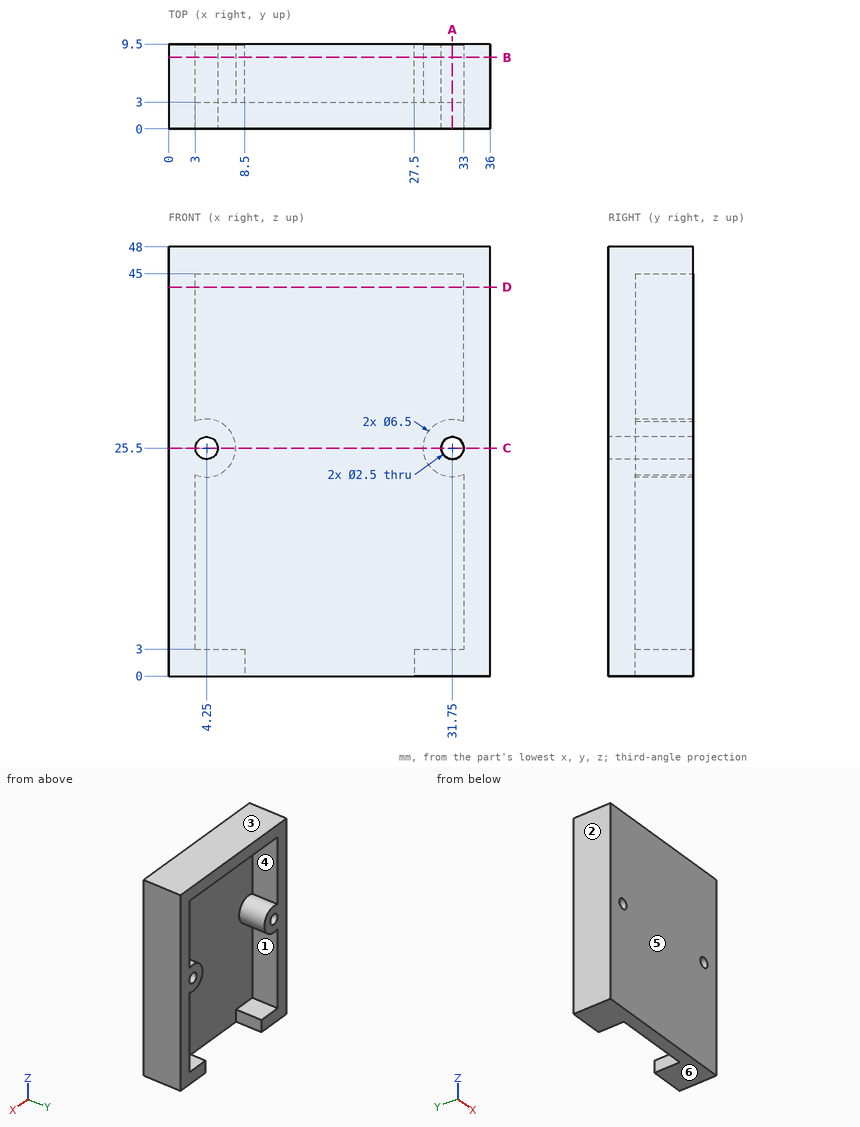
Check sheet for the drawn part. Datum: minimum x, y, z corner. Units: mm. A direction names the side the tool comes from. Coordinates: 2 decimals unless noted, no trailing zeros. Order: outer loops, then holes, each group sorted by start corner. A loop starts at its lowest first (then second) coordinate and runs counter-clockwise, first axis right, second up. Notation, with made-up numbers: (55, 1) -> (114, 1) arc R25 cw to (114, 21) -> close; hole circle Ø4 at (19.5, 9.25). An arc over 180 degrees is marked (long way). Write each question's results on one line, items separated by ' | '. Start each with the question number.
1) Section check B-B (y = 8). Enter the section's corners in (x, z), and give its area (3 significant figures).
2) Set-up check for the marked faces 1 and 2: record each of +Z, -Z, +X, -X, +Y, -Y from which the full face is reachable in a straight line by a thin tool's end or side.
3) Draft check along Z on the marked faces 3, 4, 5 and 6. Enter one of: pulls with the +Z half, pulls with the -Z half, needs draft (parallel to the pull), parting line crosses it, or undercut.
4) Material ranges on line 1 along Z through (x, y) = (31.75, 5); line 2 along X through (y, z) = (3.75, 43); line 3 along X through (y, z) = (7.75, 26.5), recorded low to high.
5) Depth check by flat-ended pin: pin 1 (3 mm diameter, centred on x = 22, y = 7.5, fed in from -Z). Enter the tip coordinate at first touch or a pass-through.
6) Section check C-C (z = 25.5). Enter the section's corners in (x, y).
7) Section check D-D (z = 43.5). Enter the section's corners in (x, y).
8) Section check A-A (x = 31.75). Enter the section's corners in (y, z).
Checked values:
1) outline: (0, 0) -> (8.5, 0) -> (8.5, 3) -> (3, 3) -> (3, 22.5) arc R3.25 ccw (long way) to (3, 28.5) -> (3, 45) -> (33, 45) -> (33, 28.5) arc R3.25 ccw (long way) to (33, 22.5) -> (33, 3) -> (27.5, 3) -> (27.5, 0) -> (36, 0) -> (36, 48) -> (0, 48) -> close; hole circle Ø2.5 at (4.25, 25.5); hole circle Ø2.5 at (31.75, 25.5) | area: 450 mm²
2) face 1: +Y | face 2: +Z, -Z, -X, +Y, -Y
3) face 3: pulls with the +Z half | face 4: undercut | face 5: needs draft | face 6: pulls with the -Z half
4) line 1: 0 to 3, 22.25 to 24.25, 26.75 to 28.75, 45 to 48 | line 2: 0 to 3, 33 to 36 | line 3: 0 to 3.5, 5 to 7.34, 28.66 to 31, 32.5 to 36
5) pin 1: z = 45
6) outline: (0, 0) -> (3, 0) -> (3, 9.5) -> (0, 9.5) -> close; (5.5, 0) -> (30.5, 0) -> (30.5, 9.5) -> (28.5, 9.5) -> (28.5, 3) -> (7.5, 3) -> (7.5, 9.5) -> (5.5, 9.5) -> close; (33, 0) -> (36, 0) -> (36, 9.5) -> (33, 9.5) -> close
7) outline: (0, 0) -> (36, 0) -> (36, 9.5) -> (33, 9.5) -> (33, 3) -> (3, 3) -> (3, 9.5) -> (0, 9.5) -> close
8) outline: (0, 0) -> (9.5, 0) -> (9.5, 3) -> (3, 3) -> (3, 22.25) -> (9.5, 22.25) -> (9.5, 24.25) -> (0, 24.25) -> close; (0, 26.75) -> (9.5, 26.75) -> (9.5, 28.75) -> (3, 28.75) -> (3, 45) -> (9.5, 45) -> (9.5, 48) -> (0, 48) -> close
